from build123d import *

# Parameters (mm, degrees)
SKETCH_1_R          = 1.25
SKETCH_1_R_2        = 5
EXTRUDE_1_DEPTH     = 5
SKETCH_2_W          = 30
SKETCH_2_H          = 30
EXTRUDE_2_DEPTH     = 9.5
SKETCH_3_R          = 5
CUT_EXTRUDE_1_DEPTH = 9.5


with BuildPart() as part:
    # 草图1 → 凸台-拉伸1 (new body)
    with BuildSketch(Plane.XY):
        with BuildLine():
            Line((0, 125), (25, 125))
            Line((25, 125), (25, -125))
            Line((25, -125), (0, -125))
            ThreePointArc((0, -125), (-125, 0), (0, 125))
        make_face()
        with Locations((0, 112.5)):
            Circle(SKETCH_1_R, mode=Mode.SUBTRACT)
        with Locations((0, 87.5)):
            Circle(SKETCH_1_R, mode=Mode.SUBTRACT)
        with Locations(Location((0, -87.5, 0), (0, 0, 180))):
            Circle(SKETCH_1_R, mode=Mode.SUBTRACT)
        with Locations(Location((0, -112.5, 0), (0, 0, 180))):
            Circle(SKETCH_1_R, mode=Mode.SUBTRACT)
        with Locations((-75, -60)):
            Circle(SKETCH_1_R_2, mode=Mode.SUBTRACT)
    extrude(amount=EXTRUDE_1_DEPTH)

    # 草图2 → 凸台-拉伸2 (add)
    with BuildSketch(Plane.XY.offset(5)):
        with Locations((-75, -60)):
            Rectangle(SKETCH_2_W, SKETCH_2_H)
    extrude(amount=EXTRUDE_2_DEPTH)

    # 草图3 → 切除-拉伸1 (cut)
    with BuildSketch(Plane(origin=(0, 0, 5), x_dir=(-1, 0, 0), z_dir=(0, 0, -1))):
        with Locations((75, -60)):
            Circle(SKETCH_3_R)
    extrude(amount=-CUT_EXTRUDE_1_DEPTH, mode=Mode.SUBTRACT)


solid = part.part
Design review of the part built by this model. Coordinates are the model's own, in mm. A direction names the side the tool comes from. Coordinates: 2 decimals unless noted, no trailing zeros. Write each loop counter-clockwise with the first axis right and the second up, starting at its lowest first coordinate (ties: lowest second). Pieces come first, ordered by that corner, then holes. Notation, with made-up numbers: (-10.75, 28) - (44.25, 28) arc R23 ccw to (44.25, 59) - close; hole circle Ø7 at (9.25, 56.25). An arc over 180 degrees is marked (long way). One line per item, written item: value.
1) For faces 4 (the face through (-75, -45, 10)), 5 (the face through (-32, 2, 0)), list the 3-axis set-ups (+Z, -Z, +X, -X, +Y, -Y) from which the entire face can be reached by the end or side of a thin tool; tool diameter is ignored.
Answer sheet:
face 4: +Z, +X, -X, +Y
face 5: -Z, +X, -X, +Y, -Y
2) Insertion check: pin 1 (2 mm diameter, centred on x = 0, y = 87.5, fed in from -Z); pin 2 (7.5 mm diameter, centred on x = -75.5, z = 9.5, fed in from -Y); pin 3 (5 mm diameter, centred on x = -3, y = 16, fed in from +Z); pin 4 (7.5 mm diameter, centred on y = -57, z = 10.5, fed in from +X). Each pin has a flat end and moves straight along its axis. Give the tip position at first contact, or say it passes through.
Answer sheet:
pin 1: passes through
pin 2: stops at y = -75
pin 3: stops at z = 5
pin 4: stops at x = -60
3) Add section B-B (z = 2.75). State the section outline as (x, y) points, plus the area to 3 significant figures.
Answer sheet:
outline: (0, -125) - (25, -125) - (25, 125) - (0, 125) arc R125 ccw to start; hole circle Ø10 at (-75, -60); hole circle Ø2.5 at (0, -112.5); hole circle Ø2.5 at (0, -87.5); hole circle Ø2.5 at (0, 87.5); hole circle Ø2.5 at (0, 112.5)
area: 30,700 mm2
4) Add section D-D (y = 0). State the section outline as (x, z) points, plus the area to 3 significant figures.
Answer sheet:
outline: (-125, 0) - (25, 0) - (25, 5) - (-125, 5) - close
area: 750 mm2
5) Add section C-C (y = -60). State the section outline as (x, z) points.
Answer sheet:
outline: (-109.66, 0) - (-80, 0) - (-80, 14.5) - (-90, 14.5) - (-90, 5) - (-109.66, 5) - close; (-70, 0) - (25, 0) - (25, 5) - (-60, 5) - (-60, 14.5) - (-70, 14.5) - close
6) Add section A-A (x = -75). State the section outline as (y, z) points.
Answer sheet:
outline: (-100, 0) - (-65, 0) - (-65, 14.5) - (-75, 14.5) - (-75, 5) - (-100, 5) - close; (-55, 0) - (100, 0) - (100, 5) - (-45, 5) - (-45, 14.5) - (-55, 14.5) - close
7) Mouldability with a two-part tool opening along X and no side actions: class faces 1 (the face through (-60, -60, 10)), 2 (the face through (-90, -60, 10)), 3 (the face through (-75, -75, 10)) as +X half, -X half, draft (parallel to the pull), parting line (faces both ways), or undercut.
Answer sheet:
face 1: +X half
face 2: -X half
face 3: draft
8) To check wall thickness, follow probe 1 along Y at (x, z) = (0, 2.45); probe 2 along Y at (x, z) = (-75, 8.5); probe 3 along Y at (x, z) = (-0.5, 0.5). State the ranges of each line that lie inside material, in increasing order.
Answer sheet:
probe 1: y = -125 to -113.75, -111.25 to -88.75, -86.25 to 86.25, 88.75 to 111.25, 113.75 to 125
probe 2: y = -75 to -65, -55 to -45
probe 3: y = -125 to -113.65, -111.35 to -88.65, -86.35 to 86.35, 88.65 to 111.35, 113.65 to 125
